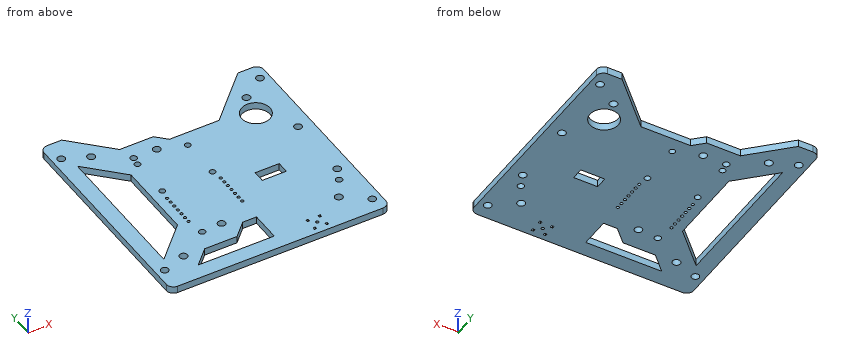
```python
from build123d import *

# Parameters (mm, degrees)
SKETCH1_W           = 92.97433
SKETCH1_H           = 93
BOSS_EXTRUDE1_DEPTH = 3
FILLET1_R           = 3
CUT_EXTRUDE1_DEPTH  = 3
SKETCH3_R           = 1.6
SKETCH3_R_2         = 1.65
SKETCH3_R_3         = 1.375
CUT_EXTRUDE2_DEPTH  = 3
SKETCH4_R           = 1.6
SKETCH4_R_2         = 1.65
SKETCH4_R_3         = 1.375
CUT_EXTRUDE3_DEPTH  = 3
SKETCH5_R           = 1.25
SKETCH5_R_2         = 0.6
CUT_EXTRUDE4_DEPTH  = 66.820259113
SKETCH2_3_W         = 10.17
SKETCH2_3_H         = 5.05
SKETCH2_3_W_2       = 1.02
SKETCH2_3_H_2       = 1.02
CUT_EXTRUDE5_DEPTH  = 10
SKETCH7_R           = 6
CUT_EXTRUDE6_DEPTH  = 66.820259113


with BuildPart() as part:
    # Sketch1 → Boss-Extrude1 (new body)
    with BuildSketch(Plane.XY):
        Rectangle(SKETCH1_W, SKETCH1_H)
    extrude(amount=BOSS_EXTRUDE1_DEPTH)

    # Fillet1
    fillet1_edges = [part.edges().sort_by_distance(p)[0] for p in [
        (46.487165, -46.5, 1.5),
        (-46.487165, -46.5, 1.5),
        (-46.487165, 46.5, 1.5),
        (46.487165, 46.5, 1.5),
    ]]
    fillet(fillet1_edges, radius=FILLET1_R)

    # Sketch2 → Cut-Extrude1 (cut)
    with BuildSketch(Plane.XY.offset(3)):
        Polygon((-39.987165, 30.80761), (-39.987165, -30.80761), (-25.722107704, -16.54254623), (-25.722107704, 16.54254623), align=None)
        Polygon((-37.295165, 46.5), (-21.908517975, 31.113359908), (-7.648517975, 31.113359908), (-3.384663123, 26.849506978), (17.674350896, 26.849506978), (37.324835, 46.5), align=None)
        Polygon((-24.13996688, -33.24619021), (-30.87162192, -39.977848283), (1.328948971, -39.977593006), (1.328948971, -27.320634039), (-4.514413398, -27.320634039), (-10.43996688, -33.24619021), align=None)
    extrude(amount=-CUT_EXTRUDE1_DEPTH, mode=Mode.SUBTRACT)

    # Sketch3 → Cut-Extrude2 (cut)
    with BuildSketch(Plane.XY.offset(3)):
        with Locations((-42.887165, 37.38)):
            Circle(SKETCH3_R)
        with Locations((-32.877165, 32.89)):
            Circle(SKETCH3_R_2)
        with Locations((-19.987165, 24.3)):
            Circle(SKETCH3_R_3)
        with Locations((-10.187165, 24.3)):
            Circle(SKETCH3_R)
    extrude(amount=-CUT_EXTRUDE2_DEPTH, mode=Mode.SUBTRACT)

    # Sketch4 → Cut-Extrude3 (cut)
    with BuildSketch(Plane.XY.offset(3)):
        with Locations((42.777165, -40.07)):
            Circle(SKETCH4_R)
        with Locations((32.877165, -32.89)):
            Circle(SKETCH4_R_2)
        with Locations((37.987165, -24.5)):
            Circle(SKETCH4_R_3)
        with Locations((40.587165, -18.8)):
            Circle(SKETCH4_R)
        with Locations((-42.887165, -36.27)):
            Circle(SKETCH4_R)
        with Locations((-32.877165, -32.89)):
            Circle(SKETCH4_R_2)
        with Locations((-19.987165, -24.5)):
            Circle(SKETCH4_R_3)
        with Locations((-11.487165, -24)):
            Circle(SKETCH4_R)
        with Locations((42.777165, 39.9)):
            Circle(SKETCH4_R)
        with Locations((32.877165, 32.89)):
            Circle(SKETCH4_R_2)
        with Locations((40.587165, 9.1)):
            Circle(SKETCH4_R)
    extrude(amount=-CUT_EXTRUDE3_DEPTH, mode=Mode.SUBTRACT)

    # Sketch5 → Cut-Extrude4 (cut, through all)
    with BuildSketch(Plane.XY.offset(3)):
        with Locations((0.691290951, 20.56)):
            Circle(SKETCH5_R)
        with Locations((-20.598709049, 20.56)):
            Circle(SKETCH5_R)
        with Locations((0.691290951, 2.9)):
            Circle(SKETCH5_R)
        with Locations((-20.598709049, 2.9)):
            Circle(SKETCH5_R)
        with Locations((-21.228709049, -1.6)):
            Circle(SKETCH5_R_2)
        with Locations((-21.228709049, -4.15)):
            Circle(SKETCH5_R_2)
        with Locations((-21.228709049, -6.7)):
            Circle(SKETCH5_R_2)
        with Locations((-21.228709049, -9.25)):
            Circle(SKETCH5_R_2)
        with Locations((-21.228709049, -11.8)):
            Circle(SKETCH5_R_2)
        with Locations((-21.228709049, -14.35)):
            Circle(SKETCH5_R_2)
        with Locations((-21.228709049, -16.9)):
            Circle(SKETCH5_R_2)
        with Locations((1.471290951, -1.6)):
            Circle(SKETCH5_R_2)
        with Locations((1.471290951, -4.15)):
            Circle(SKETCH5_R_2)
        with Locations((1.471290951, -6.7)):
            Circle(SKETCH5_R_2)
        with Locations((1.471290951, -9.25)):
            Circle(SKETCH5_R_2)
        with Locations((1.471290951, -11.8)):
            Circle(SKETCH5_R_2)
        with Locations((1.471290951, -14.35)):
            Circle(SKETCH5_R_2)
        with Locations((1.471290951, -16.9)):
            Circle(SKETCH5_R_2)
    extrude(amount=-CUT_EXTRUDE4_DEPTH, mode=Mode.SUBTRACT)

    # Sketch2<3> → Cut-Extrude5 (cut)
    with BuildSketch(Plane.XY.offset(3)):
        with Locations((18.862165, -7.995)):
            Rectangle(SKETCH2_3_W, SKETCH2_3_H)
        with Locations((16.322165, -38.61)):
            Rectangle(SKETCH2_3_W_2, SKETCH2_3_H_2)
        with Locations((21.402165, -38.61)):
            Rectangle(SKETCH2_3_W_2, SKETCH2_3_H_2)
        with BuildLine():
            ThreePointArc((19.502165, -41.15), (19.31471334, -40.69745166), (18.862165, -40.51))
            Line((18.862165, -40.51), (18.862165, -41.15))
            Line((18.862165, -41.15), (19.502165, -41.15))
        make_face()
        with BuildLine():
            Line((18.862165, -41.15), (18.862165, -40.51))
            ThreePointArc((18.862165, -40.51), (18.40961666, -40.69745166), (18.222165, -41.15))
            Line((18.222165, -41.15), (18.862165, -41.15))
        make_face()
        with BuildLine():
            Line((19.502165, -41.15), (18.862165, -41.15))
            Line((18.862165, -41.15), (18.862165, -41.79))
            ThreePointArc((18.862165, -41.79), (19.31471334, -41.60254834), (19.502165, -41.15))
        make_face()
        with BuildLine():
            Line((18.862165, -41.79), (18.862165, -41.15))
            Line((18.862165, -41.15), (18.222165, -41.15))
            ThreePointArc((18.222165, -41.15), (18.40961666, -41.60254834), (18.862165, -41.79))
        make_face()
        with Locations((21.402165, -43.69)):
            Rectangle(SKETCH2_3_W_2, SKETCH2_3_H_2)
        with Locations((16.322165, -43.69)):
            Rectangle(SKETCH2_3_W_2, SKETCH2_3_H_2)
    extrude(amount=-CUT_EXTRUDE5_DEPTH, mode=Mode.SUBTRACT)

    # Sketch7 → Cut-Extrude6 (cut, through all)
    with BuildSketch(Plane.XY.offset(3)):
        with Locations((31.287165, 23.5)):
            Circle(SKETCH7_R)
    extrude(amount=-CUT_EXTRUDE6_DEPTH, mode=Mode.SUBTRACT)


solid = part.part
```
The listing builds one solid part. Answer for the finished solid, in the listing's coordinates (mm). Coordinates: 2 decimals unless noted, no trailing zeros. Loops run counter-clockwise (first coordinate to the right, second up) from the corner with the lowest first, then second, coordinate; pieces in that order, holes last. Notation, with made-up numbers: (-0.5, 11.25) - (54.5, 11.25) arc R24 ccw to (54.5, 32.25) - close; hole circle Ø10 at (68, 37). An arc over 180 degrees is marked (long way). Write item = value, one per line.
1) Section A-A (y = 20.56) is taken. Determine the outline of the cut face in (x, z), plus the area to 3 significant figures.
Responses:
outline = (-46.49, 0) - (-39.99, 0) - (-39.99, 3) - (-46.49, 3) - close; (-29.74, 0) - (-21.85, 0) - (-21.85, 3) - (-29.74, 3) - close; (-19.35, 0) - (-0.56, 0) - (-0.56, 3) - (-19.35, 3) - close; (1.94, 0) - (26.06, 0) - (26.06, 3) - (1.94, 3) - close; (36.52, 0) - (46.49, 0) - (46.49, 3) - (36.52, 3) - close
area = 202 mm^2
2) Section C-C (z = 1.5) is taken. Count the separate pieces of the cut face and the enclosed holes in it, plus the area to 3 significant figures.
Responses:
separate_pieces = 1
enclosed_holes = 42
area = 6,380 mm^2
3) Find the intervals of material crossed by line 1 along X through (y, z) = (40.5, 2.3); line 2 along X through (y, z) = (31.5, 2.65); line 3 along X through (y, z) = (7, 1.1), in increasing order.
Responses:
line_1 = -46.49 to -31.3, 31.32 to 41.29, 44.26 to 46.49
line_2 = -46.49 to -33.77, -31.99 to -22.3, 22.32 to 31.99, 33.77 to 46.49
line_3 = -46.49 to -39.99, -25.72 to 46.49
4) Each of these flat-tipped pins is pushed along its axis until it touches: P1, Ø0.9, axis at x = 20, z = 1.5, coming from the +Y side; P2, Ø4, axis at x = -32.88, y = -32.89, coming from the -Z side; P3, Ø0.8, axis at x = 16.5, z = 2, coming from the +Y side. Where does it stop, or does it pass through?
Responses:
P1 = 29.63
P2 = 0
P3 = 26.85
5) Section B-B (y = 32.89) is taken. Determine the outline of the cut face in (x, z).
Responses:
outline = (-46.49, 0) - (-34.53, 0) - (-34.53, 3) - (-46.49, 3) - close; (-31.23, 0) - (-23.69, 0) - (-23.69, 3) - (-31.23, 3) - close; (23.71, 0) - (31.23, 0) - (31.23, 3) - (23.71, 3) - close; (34.53, 0) - (46.49, 0) - (46.49, 3) - (34.53, 3) - close
6) Section D-D (y = -36.27) is taken. Determine the outline of the cut face in (x, z).
Responses:
outline = (-46.49, 0) - (-44.49, 0) - (-44.49, 3) - (-46.49, 3) - close; (-41.29, 0) - (-27.16, 0) - (-27.16, 3) - (-41.29, 3) - close; (1.33, 0) - (46.49, 0) - (46.49, 3) - (1.33, 3) - close
